```python
from build123d import *

# Parameters (mm, degrees)
SKETCH1_R           = 0.89
SKETCH1_R_2         = 1.143
BOSS_EXTRUDE1_DEPTH = 1.5875


with BuildPart() as part:
    # Sketch1 → Boss-Extrude1 (new body)
    with BuildSketch(Plane(origin=(0, 0, 0), x_dir=(1, 0, 0), z_dir=(0, 1, 0))):
        with BuildLine():
            Line((-26.7, -6.35), (26.7, -6.35))
            Line((26.7, -6.35), (26.7, 6.35))
            Line((26.7, 6.35), (-1.3, 6.35))
            add(Edge.make_bspline(
                [(-26.7, 2.65), (-1.3, 2.65), (-1.3, 6.35)],
                knots=[4.71238898, 4.71238898, 4.71238898, 6.283185307, 6.283185307, 6.283185307], degree=2, weights=[1, 0.707106781, 1]))
            Line((-26.7, 2.65), (-30.7, 2.65))
            Line((-30.7, 2.65), (-30.7, -6.35))
            Line((-30.7, -6.35), (-26.7, -6.35))
        make_face()
        with Locations(Location((-26.7, 0.9, 0), (0, 0, 270))):
            Circle(SKETCH1_R, mode=Mode.SUBTRACT)
        with Locations(Location((-26.7, -4.6, 0), (0, 0, 270))):
            Circle(SKETCH1_R, mode=Mode.SUBTRACT)
        with Locations(Location((2.7, 3.25, 0), (0, 0, 270))):
            Circle(SKETCH1_R_2, mode=Mode.SUBTRACT)
        with Locations(Location((2.7, -3.25, 0), (0, 0, 270))):
            Circle(SKETCH1_R_2, mode=Mode.SUBTRACT)
        with Locations(Location((22.7, 3.25, 0), (0, 0, 270))):
            Circle(SKETCH1_R_2, mode=Mode.SUBTRACT)
        with Locations(Location((22.7, -3.25, 0), (0, 0, 270))):
            Circle(SKETCH1_R_2, mode=Mode.SUBTRACT)
    extrude(amount=BOSS_EXTRUDE1_DEPTH)


solid = part.part
```
Here's how the part is built. I have some questions about the finished solid (model axes, mm). A direction names the side the tool comes from. Coordinates: 2 decimals unless noted, no trailing zeros. Order: outer loops, then holes, each group sorted by start corner. A loop starts at its lowest first (then second) coordinate and runs counter-clockwise, first axis right, second up. Notation, with made-up numbers: (5.25, 73.5) - (14.25, 73.5) arc R11 cw to (14.25, 89.5) - close; hole circle Ø9 at (18.25, 69.25). An arc over 180 degrees is marked (long way). One line per question, with ' | ' between items.
(1) Suppose I cut it at B-B on x = 22.7. List the corners of the cut face in (y, z) for me.
Report:
outline: (0, -6.35) - (1.59, -6.35) - (1.59, -4.39) - (0, -4.39) - close; (0, -2.11) - (1.59, -2.11) - (1.59, 2.11) - (0, 2.11) - close; (0, 4.39) - (1.59, 4.39) - (1.59, 6.35) - (0, 6.35) - close
(2) Will this pin go through, and if not, where does the flat tip stop? pin 1 (0.8 mm diameter, centred on x = -28, y = 1, fed in from -Z).
Report:
pin 1: stops at z = -2.65
(3) Suppose I cut it at A-A on z = -0.9. List the corners of the cut face in (x, y) for me.
Report:
outline: (-30.7, 0) - (-27.59, 0) - (-27.59, 1.59) - (-30.7, 1.59) - close; (-25.81, 0) - (26.7, 0) - (26.7, 1.59) - (-25.81, 1.59) - close
(4) Suppose I cut it at C-C on y = 0.9. State how many separate pieces and enclosed holes the cut face has, and give its area (3 significant figures).
Report:
separate pieces: 1 | enclosed holes: 6 | area: 619 mm2
(5) If we mould it in two halves opening along X, with no side actions, what happens to faces 1 (the cylindrical face through (3.472, 0.783, 2.408)), 2 (the flat face through (-2, 1.588, 0)), 3 (the cylindrical face through (3.472, 0.783, -4.092)), 4 (the flat face through (-30.7, 1, 2))? For each: pulls with the +X half, pulls with the -X half, needs draft (parallel to the pull), parting line crosses it, or undercut.
Report:
face 1: undercut | face 2: needs draft | face 3: undercut | face 4: pulls with the -X half
(6) For faces 5 (the cylindrical face through (21.584, 0.783, -3.498)), 6 (the flat face through (-29, 1, -2.65)), which set-ups out of +Z, -Z, +X, -X, +Y, -Y let a thin tool reach every point of the face, with its end or its side?
Report:
face 5: +Y, -Y | face 6: -Z, -X, +Y, -Y
(7) If I drill on L1, parallel to X at y = 0.2, z = 2.5; L2, parallel to X at y = 0.5, z = 3.25; L3, parallel to X at y = 1.05, z = 4.6, over which ranges is the centre line in solid material (lowest first)?
Report:
L1: x = -30.7 to 1.84, 3.56 to 21.84, 23.56 to 26.7 | L2: x = -30.7 to 1.56, 3.84 to 21.56, 23.84 to 26.7 | L3: x = -30.7 to -27.59, -25.81 to 26.7
